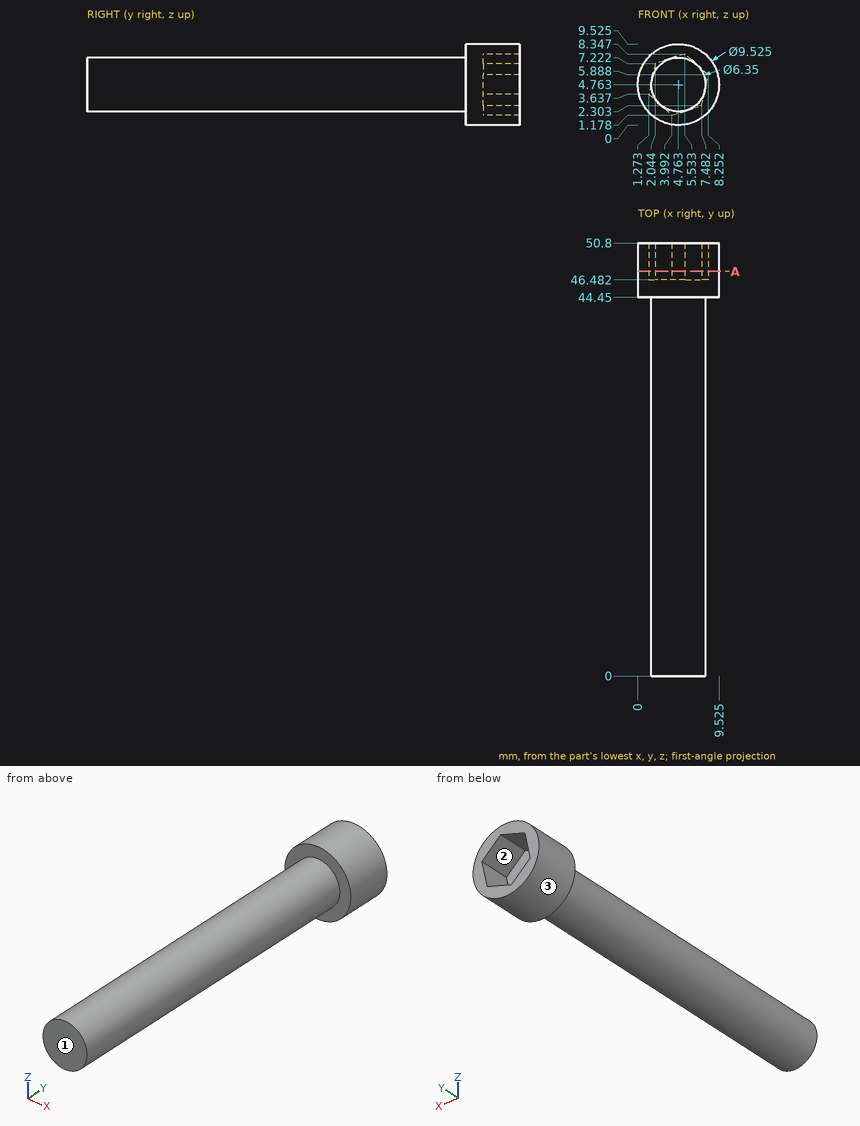
Print and shaded views of the part. All mm, measured from the part's lowest x, y and z. Give positions to 0.01 mm unless a question says otherwise; leave off trailing zeros. Write each loop counter-clockwise with the first axis right and the second up, starting at its lowest first coordinate (ties: lowest second). Pieces come first, ordered by that corner, then holes. Notation, with made-up numbers: (2.5, -3) -> (57.5, -3) arc R25 ccw to (57.5, 35) -> close; hole circle Ø1 at (0, 17.5). An arc over 180 degrees is marked (long way). Write each question's results on one line, items separated by ' | '.
1. Drop flat-ended pins along their axis: P1, Ø1, axis at y = 25.5, z = 6.5, coming from the +X side; P2, Ø4, axis at y = 13.5, z = 3.5, coming from the -X side; P3, Ø1, axis at x = 3.5, y = 10.5, coming from the +Z side (1 decimal). Give the stop position or say it passes through.
Geometry check:
P1: x = 7.69 | P2: x = 1.59 | P3: z = 7.8
2. Cut at A-A, the plane y = 47.5. Write the cut outline in (x, z) (1 decimal).
Geometry check:
outline: circle Ø9.5 at (4.8, 4.8); hole (1.3, 3.6) -> (4, 1.2) -> (7.5, 2.3) -> (8.3, 5.9) -> (5.5, 8.3) -> (2, 7.2) -> close
3. Wall check: probe 1 along Y at (x, z) = (1, 6.25); probe 2 along X at (y, z) = (15, 4.75); probe 3 along Y at (x, z) = (7.75, 4.25). Give the ranges that are in metal, low to high. Write a range as [from, to].
Geometry check:
probe 1: [44.45, 50.8] | probe 2: [1.59, 7.94] | probe 3: [0, 46.48]
4. Two-plate mould, pull along Z, no slides. Class the marked faces 1, 2 and 3: pulls with the +Z half, pulls with the -Z half, needs draft (parallel to the pull), parting line crosses it, or undercut.
Geometry check:
face 1: needs draft | face 2: undercut | face 3: parting line crosses it
